```python
from build123d import *

# Parameters (mm, degrees)
CROQUIS1_R              = 10
SALIENTE_EXTRUIR1_DEPTH = 71
CROQUIS3_W              = 0.1
CROQUIS3_H              = 30
CROQUIS4_R              = 4
SALIENTE_EXTRUIR2_DEPTH = 5
CROQUIS5_R              = 4
SALIENTE_EXTRUIR3_DEPTH = 5


with BuildPart() as part:
    # Croquis1 → Saliente-Extruir1 (new body)
    with BuildSketch(Plane(origin=(0, 0, 0), x_dir=(1, 0, 0), z_dir=(0, 1, 0))):
        Circle(CROQUIS1_R)
    extrude(amount=SALIENTE_EXTRUIR1_DEPTH)

    # Croquis3 → Cortar-Revolución1 (revolve, cut)
    with BuildSketch(Plane(origin=(0, 0, 0), x_dir=(0, 0, -1), z_dir=(1, 0, 0))):
        with Locations((9.95, 37.25)):
            Rectangle(CROQUIS3_W, CROQUIS3_H)
    revolve(axis=Axis((0, 71, 0), (0, -1, 0)), mode=Mode.SUBTRACT)

    # Croquis4 → Saliente-Extruir2 (add)
    with BuildSketch(Plane(origin=(0, 0, 0), x_dir=(-1, 0, 0), z_dir=(0, -1, 0))):
        Circle(CROQUIS4_R)
    extrude(amount=SALIENTE_EXTRUIR2_DEPTH)

    # Croquis5 → Saliente-Extruir3 (add)
    with BuildSketch(Plane(origin=(0, 71, 0), x_dir=(1, 0, 0), z_dir=(0, 1, 0))):
        Circle(CROQUIS5_R)
    extrude(amount=SALIENTE_EXTRUIR3_DEPTH)


solid = part.part
```
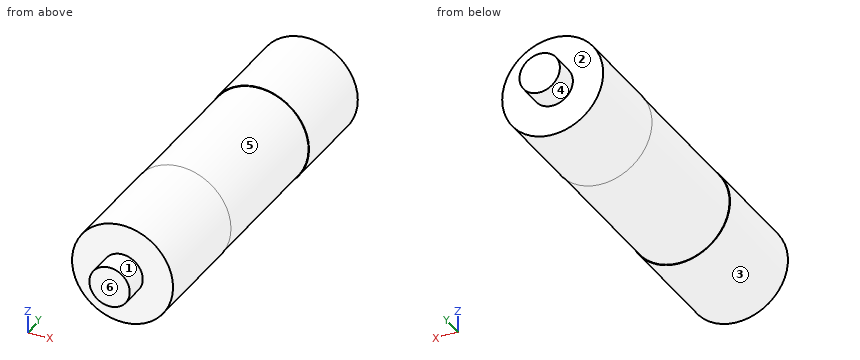
Check sheet for the modelled part. Datum: model origin and axes. Units: mm. Face numbers are marked on the shaded views. A direction names the side the tool comes from. Give positions to 0.01 mm unless a question says otherwise; leave off trailing zeros. Write each loop counter-clockwise with the first axis right and the second up, starting at its lowest first coordinate (ties: lowest second). Pieces come first, ordered by that corner, then holes. Notation, with made-up numbers: (78.5, 27.5) - (112.5, 27.5) arc R16 cw to (112.5, 55.5) - close; hole circle Ø5 at (39, -24). An arc over 180 degrees is marked (long way). Answer as a JSON object with one key per item and string values. Group by question number.
1) Sectioned sample at A-A (z = 0). Record the cut outline in (x, y).
2) Sectioned sample at B-B (x = 0). Record the cut outline in (y, z).
3) Access from +Z, -Z, +X, -X, +Y, -Y to the whole of each face (thin tool, end or side, straight path). Record for the marked faces 1, 2 and 3.
4) Sectioned sample at C-C (y = 69). Record the cut outline in (x, z).
5) Thickness scan on probe 1 along Y at (x, z) = (-4.5, -8.25); probe 2 along Z at (x, y) = (-0.5, 29.5); probe 3 along X at (y, z) = (30, -6.25). Record the ranges inside material, lowest first. Write a range as from..to.
6) Release check for a two-part mould opening along Y. For the marked faces 4, 5 and 6 record: pulls with the +Y half, pulls with the -Y half, needs draft (parallel to the pull), parting line crosses it, or undercut.
7) Sectioned sample at D-D (x = 5.75). Record the cut outline in (y, z).
8) Depth check by flat-ended pin: P1, Ø1.5, axis at x = -2.5, z = 5, coming from the +Y side; P2, Ø1.5, axis at x = 6, z = -0.5, coming from the -Y side; P3, Ø5, axis at x = -1.5, y = 36, coming from the +Z side. Enter the tip coordinate at first touch or a pass-through.
Geometry results:
{
 "1": {"outline": "(-10, 0) - (-4, 0) - (-4, -5) - (4, -5) - (4, 0) - (10, 0) - (10, 22.25) - (9.9, 22.25) - (9.9, 52.25) - (10, 52.25) - (10, 71) - (4, 71) - (4, 76) - (-4, 76) - (-4, 71) - (-10, 71) - (-10, 52.25) - (-9.9, 52.25) - (-9.9, 22.25) - (-10, 22.25) - close"},
 "2": {"outline": "(-5, -4) - (0, -4) - (0, -10) - (22.25, -10) - (22.25, -9.9) - (52.25, -9.9) - (52.25, -10) - (71, -10) - (71, -4) - (76, -4) - (76, 4) - (71, 4) - (71, 10) - (52.25, 10) - (52.25, 9.9) - (22.25, 9.9) - (22.25, 10) - (0, 10) - (0, 4) - (-5, 4) - close"},
 "3": {"face 1": "-Y", "face 2": "+Y", "face 3": "+Y, -Y"},
 "4": {"outline": "circle Ø20 at (0, 0)"},
 "5": {"probe 1": "y = 0..71", "probe 2": "z = -9.89..9.89", "probe 3": "x = -7.68..7.68"},
 "6": {"face 4": "needs draft", "face 5": "undercut", "face 6": "pulls with the -Y half"},
 "7": {"outline": "(0, -8.18) - (22.25, -8.18) - (22.25, -8.06) - (52.25, -8.06) - (52.25, -8.18) - (71, -8.18) - (71, 8.18) - (52.25, 8.18) - (52.25, 8.06) - (22.25, 8.06) - (22.25, 8.18) - (0, 8.18) - close"},
 "8": {"P1": "stops at y = 71", "P2": "stops at y = 0", "P3": "stops at z = 9.9"}
}
